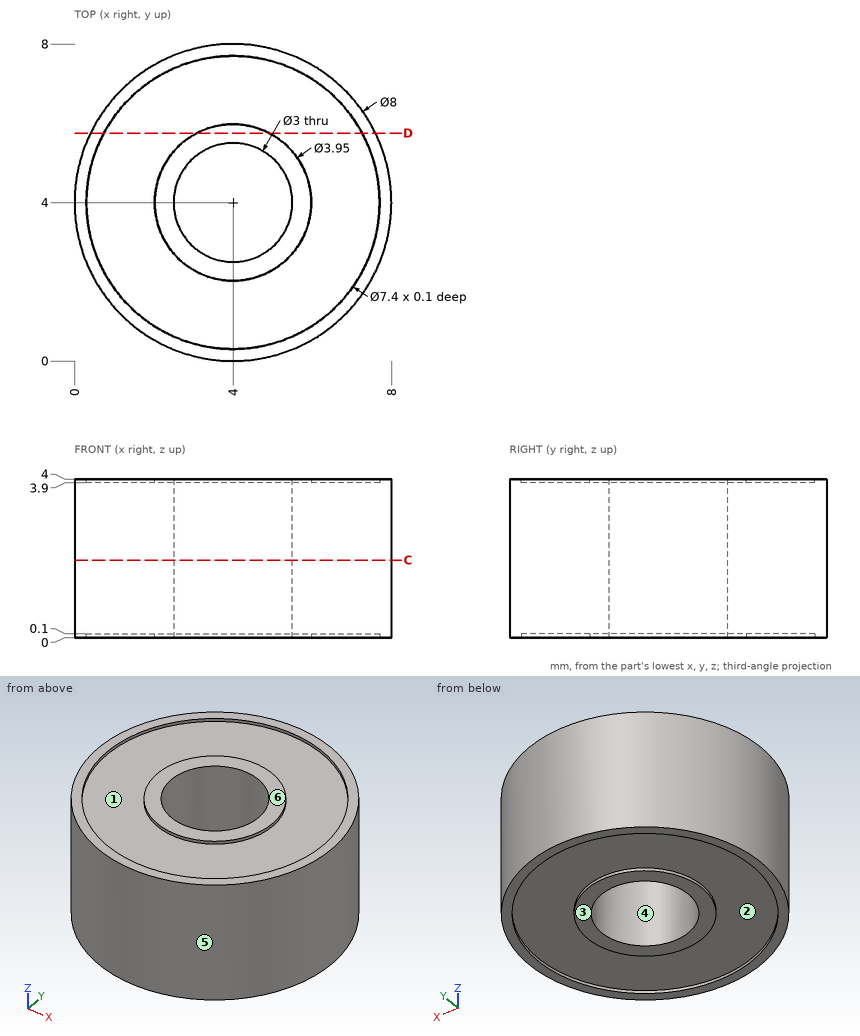
Check sheet for the drawn part. Datum: minimum x, y, z corner. Units: mm. A direction names the side the tool comes from. Give positions to 0.01 mm unless a question says otherwise; leave off trailing zeros. Write each loop counter-clockwise with the first axis right and the second up, starting at its lowest first coordinate (ties: lowest second). Pieces come first, ordered by that corner, then holes. Notation, with made-up numbers: M 10,27 L 32,27 A20 cw 32,62 Z; hole C -37.75,32 d6. An arc over 180 degrees is marked long. One line per question, with ' | ' between items.
1) Mould release check, pull along X, two halves, no side actions. Record for the marked faces 4, 5 and 6: released by +X, released by -X, zero draft, split by the parting line, or undercut.
Result:
face 4: undercut | face 5: split by the parting line | face 6: zero draft
2) Section check D-D on y = 5.75. Enter the section's corners in (x, z).
Result:
outline: M 0.4,0 L 0.74,0 L 0.74,0.1 L 3.08,0.1 L 3.08,0 L 4.92,0 L 4.92,0.1 L 7.26,0.1 L 7.26,0 L 7.6,0 L 7.6,4 L 7.26,4 L 7.26,3.9 L 4.92,3.9 L 4.92,4 L 3.08,4 L 3.08,3.9 L 0.74,3.9 L 0.74,4 L 0.4,4 Z
3) Section check C-C on z = 1.95. Enter the section's corners in (x, y).
Result:
outline: C 4,4 d8; hole C 4,4 d3
4) Thickness scan on line 1 along Y through (x, z) = (4, 3.95) (1 decimal); line 2 along Y through (x, z) = (4, 0.8); line 3 along Z through (x, y) = (1.5, 5.25). Record the ranges inside material, lowest first. Write a range as [from, to].
Result:
line 1: y = [0, 0.3], [2, 2.5], [5.5, 6], [7.7, 8] | line 2: y = [0, 2.5], [5.5, 8] | line 3: z = [0.1, 3.9]
5) Gauge pin test, flat end, axial feed: pin 1 Ø1.5 at (y, z) = (6, 3.5) entering from -X. Record the tip position at first contact, or that the pin passes through.
Result:
pin 1: stops at x = 0.2
6) Set-up check for the marked faces 1, 2 and 3: record each of +Z, -Z, +X, -X, +Y, -Y from which the full face is reachable in a straight line by a thin tool's end or side.
Result:
face 1: +Z | face 2: -Z | face 3: -Z, +X, -X, +Y, -Y
